CAD build for the part. Positions are in the model's coordinates, mm. Face numbers are marked on the shaded views. A direction names the side the tool comes from. Give positions to 0.01 mm unless a question says otherwise; leave off trailing zeros. Loops run counter-clockwise (first coordinate to the right, second up) from the corner with the lowest first, then second, coordinate; pieces in that order, holes last. Notation, with made-up numbers: M 81.5,89.25 L 128.5,89.25 A19 cw 128.5,99.25 Z; hole C 32.5,-3 d1. An arc over 180 degrees is marked long. One line per question, with ' | ' between items.
```python
from build123d import *

# Parameters (mm, degrees)
RESSALTO_EXTRUS_O1_DEPTH = 3.15
ESBO_O2_OUTSIDE_W        = 11.52
ESBO_O2_OUTSIDE_H        = 6.47
CORTE_EXTRUS_O1_DEPTH    = 3.5


with BuildPart() as part:
    # Esboço1 → Ressalto-extrusão1 (new, symmetric)
    with BuildSketch(Plane.XY):
        with BuildLine():
            Line((3.2, 1.225), (-3.2, 1.225))
            ThreePointArc((-3.2, 1.225), (-3.58890873, 1.06390873), (-3.75, 0.675))
            Line((-3.75, 0.675), (-3.75, 0.157817459))
            ThreePointArc((-3.75, 0.157817459), (-3.708133743, -0.052658428), (-3.58890873, -0.23109127))
            Line((-3.58890873, -0.23109127), (-2.75609127, -1.06390873))
            ThreePointArc((-2.75609127, -1.06390873), (-2.577658428, -1.183133743), (-2.367182541, -1.225))
            Line((-2.367182541, -1.225), (2.367182541, -1.225))
            ThreePointArc((2.367182541, -1.225), (2.577658428, -1.183133743), (2.75609127, -1.06390873))
            Line((2.75609127, -1.06390873), (3.58890873, -0.23109127))
            ThreePointArc((3.58890873, -0.23109127), (3.708133743, -0.052658428), (3.75, 0.157817459))
            Line((3.75, 0.157817459), (3.75, 0.675))
            ThreePointArc((3.75, 0.675), (3.58890873, 1.06390873), (3.2, 1.225))
        make_face()
    extrude(amount=RESSALTO_EXTRUS_O1_DEPTH, both=True)

    # Esboço2 outside → Corte-extrusão1 (cut)
    # profile 1 of 2: a face of its own
    with BuildSketch(Plane.XY.offset(3.15)):
        Rectangle(ESBO_O2_OUTSIDE_W, ESBO_O2_OUTSIDE_H)
        with BuildLine():
            Line((2.75609127, -1.06390873), (3.58890873, -0.23109127))
            ThreePointArc((3.58890873, -0.23109127), (3.708133743, -0.052658428), (3.75, 0.157817459))
            Line((3.75, 0.157817459), (3.75, 0.675))
            ThreePointArc((3.75, 0.675), (3.58890873, 1.06390873), (3.2, 1.225))
            Line((3.2, 1.225), (-3.2, 1.225))
            ThreePointArc((-3.2, 1.225), (-3.58890873, 1.06390873), (-3.75, 0.675))
            Line((-3.75, 0.675), (-3.75, 0.157817459))
            ThreePointArc((-3.75, 0.157817459), (-3.708133743, -0.052658428), (-3.58890873, -0.23109127))
            Line((-3.58890873, -0.23109127), (-2.75609127, -1.06390873))
            ThreePointArc((-2.75609127, -1.06390873), (-2.577658428, -1.183133743), (-2.367182541, -1.225))
            Line((-2.367182541, -1.225), (2.367182541, -1.225))
            ThreePointArc((2.367182541, -1.225), (2.577658428, -1.183133743), (2.75609127, -1.06390873))
        make_face(mode=Mode.SUBTRACT)
    # profile 2 of 2: a face of its own
    with BuildSketch(Plane.XY.offset(3.15)):
        with BuildLine():
            Line((-3.45, 0.675), (-3.45, 0.157817459))
            ThreePointArc((-3.45, 0.157817459), (-3.430969883, 0.062146601), (-3.376776695, -0.018959236))
            Line((-3.376776695, -0.018959236), (-2.543959236, -0.851776695))
            ThreePointArc((-2.543959236, -0.851776695), (-2.462853399, -0.905969883), (-2.367182541, -0.925))
            Line((-2.367182541, -0.925), (2.367182541, -0.925))
            ThreePointArc((2.367182541, -0.925), (2.462853399, -0.905969883), (2.543959236, -0.851776695))
            Line((2.543959236, -0.851776695), (3.376776695, -0.018959236))
            ThreePointArc((3.376776695, -0.018959236), (3.430969883, 0.062146601), (3.45, 0.157817459))
            Line((3.45, 0.157817459), (3.45, 0.675))
            ThreePointArc((3.45, 0.675), (3.376776695, 0.851776695), (3.2, 0.925))
            Line((3.2, 0.925), (-3.2, 0.925))
            ThreePointArc((-3.2, 0.925), (-3.376776695, 0.851776695), (-3.45, 0.675))
        make_face()
    extrude(amount=-CORTE_EXTRUS_O1_DEPTH, mode=Mode.SUBTRACT)


solid = part.part
```
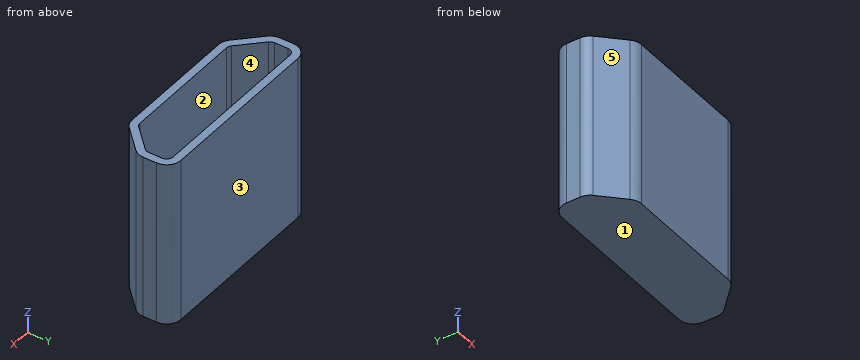
Item 1: Drop a flat-ended pin along its axis: P1, Ø1, axis at x = 3, y = 0, coming from the +Z side. Give the stop position or say it passes through.
Conclusion:
P1: z = 3.15
Item 2: Saw through at A-A on y = 0.55. Give the cut face in (x, z).
Conclusion:
outline: M -3.75,-3.15 L 3.75,-3.15 L 3.75,3.15 L 3.45,3.15 L 3.45,-0.35 L -3.45,-0.35 L -3.45,3.15 L -3.75,3.15 Z
Item 3: Saw through at C-C on x = 1.25. Give the cut face in (y, z) (3 decimals), and give its area (3 significant figures).
Conclusion:
outline: M -1.225,-3.15 L 1.225,-3.15 L 1.225,3.15 L 0.925,3.15 L 0.925,-0.35 L -0.925,-0.35 L -0.925,3.15 L -1.225,3.15 Z | area: 8.96 mm²
Item 4: Mould opens along X. For the marked faces 3, 4 and 5 say: pulls with the +X half, pulls with the -X half, needs draft (parallel to the pull), parting line crosses it, or undercut.
Conclusion:
face 3: needs draft | face 4: undercut | face 5: pulls with the -X half
Item 5: Drill centre lines: line 1 along X through (y, z) = (0.2, 0.5); line 2 along Y through (x, z) = (-1.75, -0.25) (3 decimals); line 3 along Z through (x, y) = (2.75, -0.1). Where is each one in solid material? Low to high. Write a range as [from, to].
Conclusion:
line 1: [-3.75, -3.45], [3.45, 3.75] | line 2: [-1.225, -0.925], [0.925, 1.225] | line 3: [-3.15, -0.35]
Item 6: Saw through at B-B on z = 0.5. Give the cut face in (x, y) (3 decimals).
Conclusion:
outline: M -3.75,0.158 A0.55 ccw -3.589,-0.231 L -2.756,-1.064 A0.55 ccw -2.367,-1.225 L 2.367,-1.225 A0.55 ccw 2.756,-1.064 L 3.589,-0.231 A0.55 ccw 3.75,0.158 L 3.75,0.675 A0.55 ccw 3.2,1.225 L -3.2,1.225 A0.55 ccw -3.75,0.675 Z; hole M -3.45,0.158 A0.25 ccw -3.377,-0.019 L -2.544,-0.852 A0.25 ccw -2.367,-0.925 L 2.367,-0.925 A0.25 ccw 2.544,-0.852 L 3.377,-0.019 A0.25 ccw 3.45,0.158 L 3.45,0.675 A0.25 ccw 3.2,0.925 L -3.2,0.925 A0.25 ccw -3.45,0.675 Z
Item 7: 3-axis set-ups, long thin cutter, end or side, ignore diameter. For the marked faces 1 and 2: which of +Z, -Z, +X, -X, +Y, -Y reach the whole face in a straight line?
Conclusion:
face 1: -Z, +X, -X, +Y, -Y | face 2: +Z
Item 8: Saw through at D-D on z = -0.5. Give the cut face in (x, y) (3 decimals).
Conclusion:
outline: M -3.75,0.158 A0.55 ccw -3.589,-0.231 L -2.756,-1.064 A0.55 ccw -2.367,-1.225 L 2.367,-1.225 A0.55 ccw 2.756,-1.064 L 3.589,-0.231 A0.55 ccw 3.75,0.158 L 3.75,0.675 A0.55 ccw 3.2,1.225 L -3.2,1.225 A0.55 ccw -3.75,0.675 Z
